Input: part model. Units: mm. Frame: model coordinates. Face numbers are marked on the shaded views. A direction names the side the tool comes from. Give positions to 0.01 mm unless a question says otherwise; leave off trailing zeros. Write each loop counter-clockwise with the first axis right and the second up, starting at its lowest first coordinate (ties: lowest second). Pieces come first, ordered by that corner, then holes.
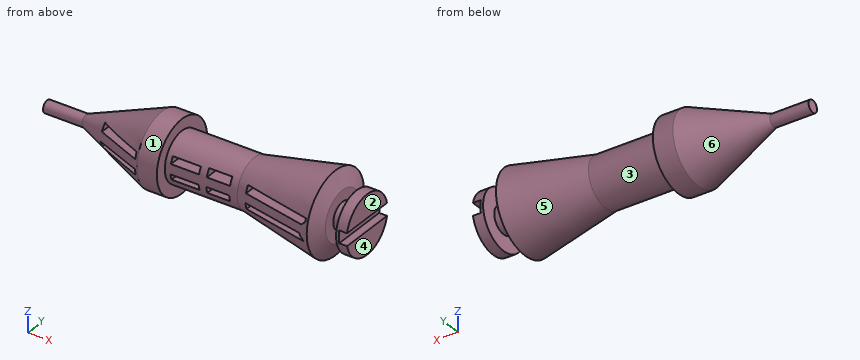
```python
from build123d import *

# Parameters (mm, degrees)
F2_W     = 30.3143421188
F2_H     = 4.0757688694
F2_W_2   = 18.1842008606
F2_W_3   = 15.0489956141
F2_H_2   = 4.7028097324
F2_W_4   = 44.4351620972
F2_H_3   = 4.4586383738
F2_W_5   = 30.713875778
F2_H_4   = 3.954576212
F2_H_5   = 3.8227577461
F2_W_6   = 14.8049108684
F2_H_6   = 4.21821489
F3_DEPTH = 25.4
F4_W     = 41.5230542421
F4_H     = 8.040972054
F5_DEPTH = 5.08


with BuildPart() as f1:
    # F0 (on Front) → F1 (revolve)
    with BuildSketch(Plane.XZ):
        Polygon((-62.0642483835, 3.9065815508), (-87.20035851, 3.9065815508), (-87.20035851, 0), (119.7071522474, 0), (119.7071522474, 18.9729742706), (112.8823459148, 18.9729742706), (112.8823459148, 8.5992645472), (103.8735955954, 8.5992645472), (103.8735955954, 15.9700587392), (99.2327257991, 26.6167614609), (46.8181893229, 15.9700587392), (0, 15.9700587392), (0, 23.3408529311), (-12.9671432078, 23.3408529311), align=None)
    revolve(axis=Axis((16.2533968687, 0, 0), (1, 0, 0)))

    # F2 (on Front) → F3 (cut)
    with BuildSketch(Plane.XZ):
        with Locations((-29.8330406658, 6.2704191078)):
            Rectangle(F2_W, F2_H)
        with Locations((12.6975956373, 6.2704191078)):
            Rectangle(F2_W_2, F2_H)
        with Locations((34.3305245042, 6.5839395393)):
            Rectangle(F2_W_3, F2_H_2)
        with Locations((75.2912443131, 6.4618538599)):
            Rectangle(F2_W_4, F2_H_3)
        with Locations((-30.0328074954, -3.7906030775)):
            Rectangle(F2_W_5, F2_H_4)
        with Locations((12.6975956373, -3.8565123104)):
            Rectangle(F2_W_2, F2_H_5)
        with Locations((34.2084821314, -3.6587837385)):
            Rectangle(F2_W_6, F2_H_6)
        with Locations((75.2912443131, -3.6587837385)):
            Rectangle(F2_W_4, F2_H_6)
    extrude(amount=F3_DEPTH, mode=Mode.SUBTRACT)

    # F4 (on face) → F5 (cut)
    with BuildSketch(Plane.YZ.offset(119.7071522474)):
        Rectangle(F4_W, F4_H)
    extrude(amount=-F5_DEPTH, mode=Mode.SUBTRACT)


solid = f1.part
```
Item 1: Section A-A (x = 33). Return loops of the section in (y, z).
Item 2: Mould query, pull axis X, two halves, no side actions, for the marked faces 4, 5 and 6. Classes: +X half, -X half, draft (parallel to the pull), parting line (faces both ways), or undercut.
Item 3: Pin query (flat end, axial travel): pin 1 (10 mm diameter, centred on x = -25.5, y = -11, fed in from -Z); pin 2 (2 mm diameter, centred on x = -22, z = 13, fed in from +Y); pin 3 (16.5 mm diameter, centred on x = 34.5, y = -8.5, fed in from +Z). Return the tip coordinate at first contact, or that it passes through.
Item 4: Ray query, line 1 (Z direction, x = 82, y = -7.5); line 2 (X direction, y = -7, z = -5.5); line 3 (Z direction, x = 97, y = -11). Return the intervals inside material, ascending.
Item 5: Set-up query: the marked faces 1, 2 and 3. Return all of +Z, -Z, +X, -X, +Y, -Y with unobstructed straight access to the full face (end or side cutting, diameter ignored); none if empty.
Item 6: Section B-B (x = -8). Return loops of the section in (y, z).
Solved:
1. outline: (-15.89, -1.55) - (0, -1.55) - (0, -5.77) - (-14.89, -5.77) arc R15.97 ccw (long way) to (-13.24, 8.94) - (0, 8.94) - (0, 4.23) - (-15.4, 4.23) arc R15.97 ccw to start
2. face 4: +X half
2. face 5: undercut
2. face 6: -X half
3. pin 1: stops at z = -18.32
3. pin 2: stops at y = 15.85
3. pin 3: stops at z = 15.97
4. line 1: z = -21.87 to -5.77, -1.55 to 4.23, 8.69 to 21.87
4. line 2: x = -49.44 to -45.39, -14.68 to 3.61, 21.79 to 26.81, 41.61 to 53.07, 97.51 to 103.87, 112.88 to 119.71
4. line 3: z = -23.74 to -5.77, -1.55 to 4.23, 8.69 to 23.74
5. face 1: -X
5. face 2: +Z, -Z, +X, +Y, -Y
5. face 3: none
6. outline: circle Ø46.68 at (0, 0)
